Part model, mm, in its own coordinate system. A direction names the side the tool comes from. Round coordinates to 2 decimals unless told otherwise and drop trailing zeros. Write each loop counter-clockwise with the first axis right and the second up, starting at its lowest first coordinate (ties: lowest second). Pieces come first, ordered by that corner, then holes.
```python
from build123d import *

# Parameters (mm, degrees)
BOSS_EXTRUDE2_DEPTH = 5
BOSS_EXTRUDE4_DEPTH = 2.5


with BuildPart() as part:
    # Sketch1 → Boss-Extrude2 (new, symmetric)
    with BuildSketch(Plane.XY):
        with BuildLine():
            Line((22, 94), (22, 124))
            ThreePointArc((22, 124), (0, 146), (-22, 124))
            Line((-22, 124), (-21.902773493, 93.124497726))
            ThreePointArc((-21.902773493, 93.124497726), (0.440442172, 73.913669144), (22, 94))
        make_face()
    extrude(amount=BOSS_EXTRUDE2_DEPTH, both=True)

    # Sketch1<7> → Boss-Extrude4 (add, symmetric)
    with BuildSketch(Plane.XY):
        with BuildLine():
            Line((28.804390709, 109.9394073), (22, 124))
            Line((22, 124), (22, 94))
            ThreePointArc((22, 94), (0.440442172, 73.913669144), (-21.902773493, 93.124497726))
            Line((-21.902773493, 93.124497726), (-22, 124))
            Line((-22, 124), (-28.804390709, 109.9394073))
            ThreePointArc((-28.804390709, 109.9394073), (-31.629698625, 91.14591256), (-23.298809999, 74.064516129))
            ThreePointArc((-23.298809999, 74.064516129), (-15.190736019, 51.78096855), (-25.79511107, 30.571428571))
            ThreePointArc((-25.79511107, 30.571428571), (0, -40), (25.79511107, 30.571428571))
            ThreePointArc((25.79511107, 30.571428571), (15.190736019, 51.78096855), (23.298809999, 74.064516129))
            ThreePointArc((23.298809999, 74.064516129), (31.629698625, 91.14591256), (28.804390709, 109.9394073))
        make_face()
        with BuildLine():
            ThreePointArc((-11.878172589, 8.294416244), (-11.969504398, 9.1450354), (-12, 10))
            ThreePointArc((-12, 10), (0, 22), (12, 10))
            ThreePointArc((12, 10), (11.969504398, 9.1450354), (11.878172589, 8.294416244))
            Line((11.878172589, 8.294416244), (10, -18))
            ThreePointArc((10, -18), (0, -28), (-10, -18))
            Line((-10, -18), (-11.878172589, 8.294416244))
        make_face(mode=Mode.SUBTRACT)
    extrude(amount=BOSS_EXTRUDE4_DEPTH, both=True)


solid = part.part
```
Q1. Cut at D-D on x = 6.5. Write the cut outline in (y, z), plus the area to 3 significant figures.
Values follow:
outline: (-39.47, -2.5) - (-25.6, -2.5) - (-25.6, 2.5) - (-39.47, 2.5) - close; (20.09, -2.5) - (74.89, -2.5) - (74.89, -5) - (145.02, -5) - (145.02, 5) - (74.89, 5) - (74.89, 2.5) - (20.09, 2.5) - close
area: 1,040 mm2
Q2. Wall check: L1, parallel to Y at x = 0, z = -0.95; L2, parallel to Z at x = -31.5, y = 24.5; L3, parallel to Y at x = -4.5, z = -2.25. Give the ranges that are in metal, low to high.
Values follow:
L1: y = -40 to -28, 22 to 146
L2: z = -2.5 to 2.5
L3: y = -39.75 to -26.93, 21.12 to 145.53
Q3. Mould opens along X. For faces 1 (the flat face through (10.952, -4.669, 0.035)), 2 (the cylindrical face through (-0.01, 73.91, 3.77)), 3 (the cylindrical face through (0, 22, 0)), 4 (the flat face through (25.45, 116.87, 0.04)) say: +X half, -X half, draft (parallel to the pull), parting line (faces both ways), or undercut.
Values follow:
face 1: undercut
face 2: parting line
face 3: undercut
face 4: +X half
Q4. Which spindle directions (+Z, -Z, +X, -X, +Y, -Y) get a long thin tool onto all of the face, cutting with end or side? Do faces 5 (the cylindrical face through (-0.01, 73.91, -3.73)), 6 (the flat face through (-10.926, -5.037, 0.035)), 7 (the flat face through (0, 110, -5)). Say none if no direction does.
Values follow:
face 5: -Z, -Y
face 6: +Z, -Z
face 7: -Z, +X, -X, +Y, -Y
Q5. Cut at C-C on y = 14.5. Write the cut outline in (x, z).
Values follow:
outline: (-37.28, -2.5) - (-11.12, -2.5) - (-11.12, 2.5) - (-37.28, 2.5) - close; (11.12, -2.5) - (37.28, -2.5) - (37.28, 2.5) - (11.12, 2.5) - close
Q6. Cut at A-A on z = -0.25. Write the cut outline in (x, y).
Values follow:
outline: (-28.8, 109.94) arc R32 ccw to (-23.3, 74.06) arc R30 cw to (-25.8, 30.57) arc R40 ccw (long way) to (25.8, 30.57) arc R30 cw to (23.3, 74.06) arc R32 ccw to (28.8, 109.94) - (22, 124) arc R22 ccw to (-22, 124) - close; hole (-11.88, 8.29) - (-10, -18) arc R10 ccw to (10, -18) - (11.88, 8.29) arc R12 ccw (long way) to start
Q7. Cut at B-B on x = -3. Write the cut outline in (y, z), plus the area to 3 significant figures.
Values follow:
outline: (-39.89, -2.5) - (-27.54, -2.5) - (-27.54, 2.5) - (-39.89, 2.5) - close; (21.62, -2.5) - (74.11, -2.5) - (74.11, -5) - (145.79, -5) - (145.79, 5) - (74.11, 5) - (74.11, 2.5) - (21.62, 2.5) - close
area: 1,040 mm2
Q8. Drop flat-ended pins along their axis: pin 1 (1 mm diameter, centred on x = -7.5, y = 35, fed in from +Z); pin 2 (2 mm diameter, centred on y = 113, z = 3, fed in from +X); pin 3 (1 mm diameter, centred on x = 4.5, y = 40.5, fed in from -Z); pin 4 (1 mm diameter, centred on y = 54, z = -4, fed in from +X). Give the stop position or say it passes through.
Values follow:
pin 1: stops at z = 2.5
pin 2: stops at x = 27.74
pin 3: stops at z = -2.5
pin 4: passes through
